```python
from build123d import *

# Parameters (mm, degrees)
F1_DEPTH = 3
F2_DEPTH = 20
F3_R     = 5


with BuildPart() as f1:
    # F0 (on Top) → F1 (new body)
    with BuildSketch(Plane.XY):
        with BuildLine():
            Line((126, -240), (126, 0))
            Line((126, 0), (123, 0))
            ThreePointArc((123, 0), (0, 123), (-123, 0))
            Line((-123, 0), (-126, 0))
            Line((-126, 0), (-126, -240))
            ThreePointArc((-126, -240), (-123.071068, -247.071068), (-116, -250))
            Line((-116, -250), (116, -250))
            ThreePointArc((116, -250), (123.071068, -247.071068), (126, -240))
        make_face()
        with BuildLine():
            Line((60, -235), (-60, -235))
            ThreePointArc((-60, -235), (-70, -225), (-60, -215))
            Line((-60, -215), (60, -215))
            ThreePointArc((60, -215), (70, -225), (60, -235))
        make_face(mode=Mode.SUBTRACT)
        with BuildLine():
            ThreePointArc((98.16313, -38), (100.16313, -40), (98.16313, -42))
            Line((98.16313, -42), (-98.16313, -42))
            ThreePointArc((-98.16313, -42), (-100.16313, -40), (-98.16313, -38))
            Line((-98.16313, -38), (98.16313, -38))
        make_face(mode=Mode.SUBTRACT)
        with BuildLine():
            ThreePointArc((-101.66612, -32), (-103.66612, -30), (-101.66612, -28))
            Line((-101.66612, -28), (101.66612, -28))
            ThreePointArc((101.66612, -28), (103.66612, -30), (101.66612, -32))
            Line((101.66612, -32), (-101.66612, -32))
        make_face(mode=Mode.SUBTRACT)
        with BuildLine():
            ThreePointArc((104.096109, -18), (106.096109, -20), (104.096109, -22))
            Line((104.096109, -22), (-104.096109, -22))
            ThreePointArc((-104.096109, -22), (-106.096109, -20), (-104.096109, -18))
            Line((-104.096109, -18), (104.096109, -18))
        make_face(mode=Mode.SUBTRACT)
        with BuildLine():
            ThreePointArc((-105.527248, -12), (-107.527248, -10), (-105.527248, -8))
            Line((-105.527248, -8), (105.527248, -8))
            ThreePointArc((105.527248, -8), (107.527248, -10), (105.527248, -12))
            Line((105.527248, -12), (-105.527248, -12))
        make_face(mode=Mode.SUBTRACT)
        with BuildLine():
            Line((106, -2), (-106, -2))
            ThreePointArc((-106, -2), (-108, 0), (-106, 2))
            Line((-106, 2), (106, 2))
            ThreePointArc((106, 2), (108, 0), (106, -2))
        make_face(mode=Mode.SUBTRACT)
        with BuildLine():
            Line((105.527248, 8), (-105.527248, 8))
            ThreePointArc((-105.527248, 8), (-107.527248, 10), (-105.527248, 12))
            Line((-105.527248, 12), (105.527248, 12))
            ThreePointArc((105.527248, 12), (107.527248, 10), (105.527248, 8))
        make_face(mode=Mode.SUBTRACT)
        with BuildLine():
            Line((104.096109, 18), (-104.096109, 18))
            ThreePointArc((-104.096109, 18), (-106.096109, 20), (-104.096109, 22))
            Line((-104.096109, 22), (104.096109, 22))
            ThreePointArc((104.096109, 22), (106.096109, 20), (104.096109, 18))
        make_face(mode=Mode.SUBTRACT)
        with BuildLine():
            Line((101.66612, 28), (-101.66612, 28))
            ThreePointArc((-101.66612, 28), (-103.66612, 30), (-101.66612, 32))
            Line((-101.66612, 32), (101.66612, 32))
            ThreePointArc((101.66612, 32), (103.66612, 30), (101.66612, 28))
        make_face(mode=Mode.SUBTRACT)
        with BuildLine():
            Line((98.16313, 38), (-98.16313, 38))
            ThreePointArc((-98.16313, 38), (-100.16313, 40), (-98.16313, 42))
            Line((-98.16313, 42), (98.16313, 42))
            ThreePointArc((98.16313, 42), (100.16313, 40), (98.16313, 38))
        make_face(mode=Mode.SUBTRACT)
        with BuildLine():
            Line((93.466572, 48), (-93.466572, 48))
            ThreePointArc((-93.466572, 48), (-95.466572, 50), (-93.466572, 52))
            Line((-93.466572, 52), (93.466572, 52))
            ThreePointArc((93.466572, 52), (95.466572, 50), (93.466572, 48))
        make_face(mode=Mode.SUBTRACT)
        with BuildLine():
            Line((87.384209, 58), (-87.384209, 58))
            ThreePointArc((-87.384209, 58), (-89.384209, 60), (-87.384209, 62))
            Line((-87.384209, 62), (87.384209, 62))
            ThreePointArc((87.384209, 62), (89.384209, 60), (87.384209, 58))
        make_face(mode=Mode.SUBTRACT)
        with BuildLine():
            Line((79.598995, 68), (-79.598995, 68))
            ThreePointArc((-79.598995, 68), (-81.598995, 70), (-79.598995, 72))
            Line((-79.598995, 72), (79.598995, 72))
            ThreePointArc((79.598995, 72), (81.598995, 70), (79.598995, 68))
        make_face(mode=Mode.SUBTRACT)
        with BuildLine():
            Line((69.541355, 78), (-69.541355, 78))
            ThreePointArc((-69.541355, 78), (-71.541355, 80), (-69.541355, 82))
            Line((-69.541355, 82), (69.541355, 82))
            ThreePointArc((69.541355, 82), (71.541355, 80), (69.541355, 78))
        make_face(mode=Mode.SUBTRACT)
        with BuildLine():
            Line((56, 88), (-56, 88))
            ThreePointArc((-56, 88), (-58, 90), (-56, 92))
            Line((-56, 92), (56, 92))
            ThreePointArc((56, 92), (58, 90), (56, 88))
        make_face(mode=Mode.SUBTRACT)
        with BuildLine():
            Line((35.156792, 98), (-35.156792, 98))
            ThreePointArc((-35.156792, 98), (-37.156792, 100), (-35.156792, 102))
            Line((-35.156792, 102), (35.156792, 102))
            ThreePointArc((35.156792, 102), (37.156792, 100), (35.156792, 98))
        make_face(mode=Mode.SUBTRACT)
        with BuildLine():
            Line((123, 0), (126, 0))
            ThreePointArc((126, 0), (0, 126), (-126, 0))
            Line((-126, 0), (-123, 0))
            ThreePointArc((-123, 0), (0, 123), (123, 0))
        make_face()
    extrude(amount=-F1_DEPTH)

    # F0 (on Top) → F2 (join)
    with BuildSketch(Plane.XY):
        with BuildLine():
            Line((123, 0), (126, 0))
            ThreePointArc((126, 0), (0, 126), (-126, 0))
            Line((-126, 0), (-123, 0))
            ThreePointArc((-123, 0), (0, 123), (123, 0))
        make_face()
    extrude(amount=F2_DEPTH)

    # F3
    f3_edges = [f1.edges().sort_by_distance(p)[0] for p in [
        (-124.5, 0, 20),
        (124.5, 0, 20),
    ]]
    fillet(f3_edges, radius=F3_R)


solid = f1.part
```
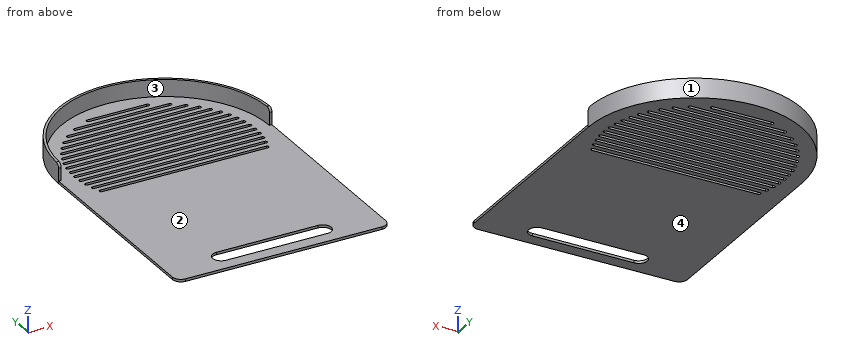
Could you check a few things on this model? Use its own coordinates, in mm. Face numbers are marked on the shaded views. Coordinates: 2 decimals unless noted, no trailing zeros. Write each loop counter-clockwise with the first axis right and the second up, starting at its lowest first coordinate (ties: lowest second). Pieces come first, ordered by that corner, then holes. Notation, with made-up numbers: (14, 15) - (48, 15) arc R28 ccw to (48, 43) - close; hole circle Ø11 at (8, 62). An arc over 180 degrees is marked (long way). Use a Markdown table: item, result.
Q1. Thinking about a two-plate mould opening in X: for the marked faces 1, 2, 3 and 4, which applies, +X half, -X half, draft (parallel to the pull), parting line (faces both ways), or undercut?
Geometry check:
| item | result |
|---|---|
| face 1 | parting line |
| face 2 | undercut |
| face 3 | undercut |
| face 4 | draft |
Q2. Imagine slicing it at A-A (z = 3.5). List the corners of the cut face in (x, y) for me.
Geometry check:
| item | result |
|---|---|
| outline | (-126, 0) - (-123, 0) arc R123 cw to (123, 0) - (126, 0) arc R126 ccw to start |
Q3. I'm going to push flat-ended pins straight in: pin 1 Ø3 at (x, y) = (-14, 40) entering from +Z; pin 2 Ø10 at (x, y) = (71, -145.5) entering from +Z; pin 3 Ø1.5 at (x, z) = (-34, -1) entering from +Y; pin 4 Ø3 at (x, z) = (11.5, 4) entering from +Y. Where does each tip first touch, or does it pass through?
Geometry check:
| item | result |
|---|---|
| pin 1 | passes through |
| pin 2 | stops at z = 0 |
| pin 3 | stops at y = 121.53 |
| pin 4 | stops at y = 125.6 |
Q4. Imagine slicing it at C-C (y = -47.5). List the corners of the cut face in (x, z) for me.
Geometry check:
| item | result |
|---|---|
| outline | (-126, -3) - (126, -3) - (126, 0) - (-126, 0) - close |
Q5. Please list where these lines run through material, in increasing order: L1, parallel to X at y = 2.5, z = 11.5; L2, parallel to Y at x = 4, z = 0.5; L3, parallel to Z at x = -32, y = -96.5.
Geometry check:
| item | result |
|---|---|
| L1 | x = -125.98 to -122.97, 122.97 to 125.98 |
| L2 | y = 122.93 to 125.94 |
| L3 | z = -3 to 0 |
Q6. Imagine slicing it at B-B (x = -52). Count the separate pieces of the cut face and the enclosed holes in it, and give its area (3 significant figures).
Geometry check:
| item | result |
|---|---|
| separate pieces | 16 |
| enclosed holes | 0 |
| area | 932 mm2 |
